Design review of the part built by this model. Coordinates are the model's own, in mm. Give positions to 0.01 mm unless a question says otherwise; leave off trailing zeros. Order: outer loops, then holes, each group sorted by start corner. A loop starts at its lowest first (then second) coordinate and runs counter-clockwise, first axis right, second up. Notation, with made-up numbers: (47.5, 33) -> (87.5, 33) arc R26 ccw to (87.5, 71) -> close; hole circle Ø6 at (58.25, -19). An arc over 180 degrees is marked (long way). One line per item, written item: value. Start each with the question number.
1) Wall thickness on line 1 along X through (y, z) = (1.45, -17); line 2 along X through (y, z) = (0.5, -10); line 3 along Z through (x, y) = (205, 0.85): over which ranges is each line inside the solid? List them lowest first. Write a range as from..to.
2) Consider section C-C (z = -60). State the section outline as (x, y) points.
3) Consider section A-A (y = 1.25). State how many separate pieces and enclosed holes the cut face has, plus the area to 3 significant figures.
4) Consider section B-B (z = -83). State the section outline as (x, y) points, plus the area to 3 significant figures.
5) The part is to be moulded in two halves that separate along X. For faces 1 (the face through (104, 2, -51)), 2 (the face through (206.669, 0.986, -90.526)), say which applies: released by +X, released by -X, zero draft, split by the parting line, or undercut.
6) Consider section D-D (x = 184). State the section outline as (y, z) points, plus the area to 3 significant figures.
from build123d import *

# Parameters (mm, degrees)
SKETCH_1_W            = 210
SKETCH_1_H            = 100
SKETCH_1_R            = 3.2
SKETCH_1_R_2          = 1.75
EXTRUDE_1_DEPTH       = 2
HOLE_WIZARD_M41_D     = 4.2
HOLE_WIZARD_M41_DEPTH = 8
HOLE_WIZARD_M41_TIP   = 1.2618073
SKETCH_4_W            = 25
SKETCH_4_H            = 3.5
CUT_EXTRUDE_1_DEPTH   = 10
FILLET_1_R            = 1


with BuildPart() as part:
    # Эскиз1 → Бобышка-Вытянуть1 (new body)
    with BuildSketch(Plane(origin=(0, 0, 0), x_dir=(1, 0, 0), z_dir=(0, 1, 0))):
        with Locations((105, 50)):
            Rectangle(SKETCH_1_W, SKETCH_1_H)
        with Locations((105, 17)):
            Circle(SKETCH_1_R, mode=Mode.SUBTRACT)
        with Locations((185, 17)):
            Circle(SKETCH_1_R, mode=Mode.SUBTRACT)
        with Locations((25, 17)):
            Circle(SKETCH_1_R, mode=Mode.SUBTRACT)
        with Locations((25, 83)):
            Circle(SKETCH_1_R, mode=Mode.SUBTRACT)
        with Locations((105, 83)):
            Circle(SKETCH_1_R, mode=Mode.SUBTRACT)
        with Locations((185, 83)):
            Circle(SKETCH_1_R, mode=Mode.SUBTRACT)
        with Locations((5, 10)):
            Circle(SKETCH_1_R_2, mode=Mode.SUBTRACT)
        with Locations((5, 90)):
            Circle(SKETCH_1_R_2, mode=Mode.SUBTRACT)
        with Locations((205, 10)):
            Circle(SKETCH_1_R_2, mode=Mode.SUBTRACT)
        with Locations((205, 90)):
            Circle(SKETCH_1_R_2, mode=Mode.SUBTRACT)
    extrude(amount=EXTRUDE_1_DEPTH)

    # Сверло под метчик  спиральное M41
    with Locations(Plane(origin=(0, 2, 0), x_dir=(1, 0, 0), z_dir=(0, 1, 0))):
        with Locations((70, 60), (140, 60), (140, 30), (70, 30)):
            Hole(HOLE_WIZARD_M41_D / 2, depth=HOLE_WIZARD_M41_DEPTH)
            with Locations((0, 0, -(HOLE_WIZARD_M41_DEPTH + HOLE_WIZARD_M41_TIP / 2))):  # 118° drill point
                Cone(0, HOLE_WIZARD_M41_D / 2, HOLE_WIZARD_M41_TIP, mode=Mode.SUBTRACT)

    # Эскиз4 → Вырез-Вытянуть1 (cut)
    with BuildSketch(Plane(origin=(0, 2, 0), x_dir=(1, 0, 0), z_dir=(0, 1, 0))):
        with Locations((105, 48.25)):
            Rectangle(SKETCH_4_W, SKETCH_4_H)
    extrude(amount=-CUT_EXTRUDE_1_DEPTH, mode=Mode.SUBTRACT)

    # Скругление1
    fillet_1_edges = [part.edges().sort_by_distance(p)[0] for p in [
        (92.5, 1, -46.5),
        (92.5, 1, -50),
        (117.5, 1, -50),
        (117.5, 1, -46.5),
    ]]
    fillet(fillet_1_edges, radius=FILLET_1_R)


solid = part.part
Checked values:
1. line 1: x = 0..21.8, 28.2..101.8, 108.2..181.8, 188.2..210
1. line 2: x = 0..3.25, 6.75..203.25, 206.75..210
1. line 3: z = -100..-91.75, -88.25..-11.75, -8.25..0
2. outline: (0, 0) -> (67.9, 0) -> (67.9, 2) -> (0, 2) -> close; (72.1, 0) -> (137.9, 0) -> (137.9, 2) -> (72.1, 2) -> close; (142.1, 0) -> (210, 0) -> (210, 2) -> (142.1, 2) -> close
3. separate pieces: 1
3. enclosed holes: 15
3. area: 20,600 mm^2
4. outline: (0, 0) -> (21.8, 0) -> (21.8, 2) -> (0, 2) -> close; (28.2, 0) -> (101.8, 0) -> (101.8, 2) -> (28.2, 2) -> close; (108.2, 0) -> (181.8, 0) -> (181.8, 2) -> (108.2, 2) -> close; (188.2, 0) -> (210, 0) -> (210, 2) -> (188.2, 2) -> close
4. area: 382 mm^2
5. face 1: zero draft
5. face 2: undercut
6. outline: (0, -100) -> (2, -100) -> (2, -86.04) -> (0, -86.04) -> close; (0, -79.96) -> (2, -79.96) -> (2, -20.04) -> (0, -20.04) -> close; (0, -13.96) -> (2, -13.96) -> (2, 0) -> (0, 0) -> close
6. area: 176 mm^2
